Autodesk Inventor part; units mm, degrees
ref_plane "YZ Plane" through (0, 0, 0) normal (1, 0, 0) x (0, 1, 0)
ref_plane "XZ Plane" through (0, 0, 0) normal (0, 1, 0) x (-1, 0, 0)
ref_plane "XY Plane" through (0, 0, 0) normal (0, 0, 1) x (1, 0, 0)
sketch "Sketch1" plane through (0, 0, 0) normal (1, 0, 0) x (0, 1, 0)
  circle A0 centre (0, 0) radius 7.1437
  circle A1 centre (0, 0) radius 19.05
  circle A2 centre (12.7, 0) radius 1.7526
  circle A3 centre (6.35, 10.9985) radius 1.7526
  circle A4 centre (-6.35, 10.9985) radius 1.7526
  circle A5 centre (-12.7, 0) radius 1.7526
  circle A6 centre (-6.35, -10.9985) radius 1.7526
  circle A7 centre (6.35, -10.9985) radius 1.7526
  dimension "d0" = 14.2875
  dimension "d1" = 38.1
  dimension "d4" = 3.5052
  dimension "d5" = 12.7
  dimension "d8" = 360
extrude "Extrusion1" add sketch "Sketch1" along normal blind 5.5563
chamfer "Chamfer1" distance 2.3813 angle 45 6 edges at (0, 10.9474, 0) (0, 4.5974, 10.9985) (0, -14.4526, 0) (0, -8.1026, 10.9985) (0, 4.5974, -10.9985) (0, -8.1026, -10.9985)
properties part number "Spacer 3-8x .125" material "UHMW, Black"
Verification items for the finished model (mm, model axes). Coordinates: 2 decimals unless noted, no trailing zeros. Order: outer loops, then holes, each group sorted by start corner. A loop starts at its lowest first (then second) coordinate and runs counter-clockwise, first axis right, second up. Notation, with made-up numbers: (-35, 19.5) -> (-1, 19.5) arc R13 ccw to (-1, 23.5) -> close; hole circle Ø3 at (-24, -22). An arc over 180 degrees is marked (long way). Use CSV: the item, a comma, the result in double quotes. Start each with the question number.
Q1. Section check C-C, the plane y = -6.35. Record the cut outline in (x, z).
Q2. Thickness scan on line 1 along Z through (x, y) = (4.45, 5.5); line 2 along Y through (x, z) = (0.75, -3); line 3 along Z through (x, y) = (1.75, 5). Record the ranges inside material, lowest first.
Q3. Depth check by flat-ended pin: P1, Ø2, axis at x = 2, y = -13.5, coming from the -Z side; P2, Ø4, axis at y = -12.7, z = 0, coming from the -X side; P3, Ø1.5, axis at x = 3.5, y = -5, coming from the +Z side; P4, Ø3, axis at y = 12.7, z = 0, coming from the -X side. Enter the tip coordinate at first touch or a pass-through.
Q4. Section check A-A, the plane z = 0. Record the cut outline in (x, y), and give its area (3 significant figures).
Q5. Section check B-B, the plane y = 0. Record the cut outline in (x, z).
Q6. Section check D-D, the plane x = 3. Record the cut outline in (y, z), and give its area (3 significant figures).
Q7. Draft check along Y on faces 1 (the cylindrical face through (3.947, -5.541, -9.444)), 2 (the flat face through (5.556, 8, 0)), 3 (the cylindrical face through (2.74, -15.12, 11.59)). Enter one of: +Y half, -Y half, draft (parallel to the pull), parting line (faces both ways), or undercut.
Returned:
1,outline,"(0, -17.96) -> (5.56, -17.96) -> (5.56, -12.75) -> (2.38, -12.75) -> (0, -15.13) -> close; (0, -6.86) -> (2.38, -9.25) -> (5.56, -9.25) -> (5.56, -3.27) -> (0, -3.27) -> close; (0, 3.27) -> (5.56, 3.27) -> (5.56, 9.25) -> (2.38, 9.25) -> (0, 6.86) -> close; (0, 15.13) -> (2.38, 12.75) -> (5.56, 12.75) -> (5.56, 17.96) -> (0, 17.96) -> close"
2,line 1,"z = -18.24 to -12.53, -9.47 to -4.56, 4.56 to 9.47, 12.53 to 18.24"
2,line 2,"y = -18.81 to -14.27, -11.13 to -6.48, 6.48 to 11.13, 14.27 to 18.81"
2,line 3,"z = -18.38 to -12.96, -9.03 to -5.1, 5.1 to 9.03, 12.96 to 18.38"
3,P1,"stops at z = -14.38"
3,P2,"stops at x = 2.13"
3,P3,"stops at z = 18.57"
3,P4,"passes through"
4,outline,"(0, -19.05) -> (5.56, -19.05) -> (5.56, -14.45) -> (2.38, -14.45) -> (0, -16.83) -> close; (0, -8.57) -> (2.38, -10.95) -> (5.56, -10.95) -> (5.56, -7.14) -> (0, -7.14) -> close; (0, 7.14) -> (5.56, 7.14) -> (5.56, 10.95) -> (2.38, 10.95) -> (0, 8.57) -> close; (0, 16.83) -> (2.38, 14.45) -> (5.56, 14.45) -> (5.56, 19.05) -> (0, 19.05) -> close"
4,area,"82.0 mm^2"
5,outline,"(0, -19.05) -> (5.56, -19.05) -> (5.56, -7.14) -> (0, -7.14) -> close; (0, 7.14) -> (5.56, 7.14) -> (5.56, 19.05) -> (0, 19.05) -> close"
6,outline,"circle Ø38.1 at (0, 0); hole circle Ø3.51 at (-12.7, 0); hole circle Ø3.51 at (-6.35, -11); hole circle Ø3.51 at (-6.35, 11); hole circle Ø14.29 at (0, 0); hole circle Ø3.51 at (6.35, -11); hole circle Ø3.51 at (6.35, 11); hole circle Ø3.51 at (12.7, 0)"
6,area,"922 mm^2"
7,face 1,"undercut"
7,face 2,"draft"
7,face 3,"parting line"
